Autodesk Inventor part; units mm, degrees
ref_plane "YZ Plane" through (0, 0, 0) normal (1, 0, 0) x (0, 1, 0)
ref_plane "XZ Plane" through (0, 0, 0) normal (0, 1, 0) x (-1, 0, 0)
ref_plane "XY Plane" through (0, 0, 0) normal (0, 0, 1) x (1, 0, 0)
sketch "Sketch1" plane through (0, 0, 0) normal (0, 0, 1) x (1, 0, 0)
  line L0 (-750, 50) -> (750, 50)
  line L1 (750, 50) -> (750, 0)
  line L2 (750, 0) -> (-750, 0)
  line L3 (-750, 0) -> (-750, 50)
  point P0 (0, 0)
  point P1 (0, 0)
  dimension "d0" = 1500
  dimension "d1" = 50
extrude "Plate1" add sketch "Sketch1" along normal blind 2
sketch "Sketch2" plane through (750, 2, 0) normal (0, -1, 0) x (1, 0, 0)
  line L0 (-1500, 0) -> (0, 0)
  line L1 (0, 0) -> (0, 30)
  line L2 (0, 30) -> (-1500, 30)
  line L3 (-1500, 30) -> (-1500, 0)
edge flange "Flange1" height 30 angle 90 thickness 2 bend radius 2.75 thickness toward (0, -1, 0) relief round relief width 2 relief depth 1 edges at (0, 0, 2) wall of the first edge with corners at (-750, 2, 0) (750, 2, 0) (750, 2, 30) (-750, 2, 30)
bend "Bend1"
corner "Corner1"
sketch "Sketch5" plane through (0, 0, 0) normal (0, 0, -1) x (-1, 0, 0)
  line L0 (750, 50) -> (-750, 50)
  line L1 (-1, 30) -> (-1, 50)
  line L2 (750, 0) -> (-750, 0)
  line L3 (-1, 30) -> (1, 30)
  line L4 (1, 30) -> (1, 50)
  point P0 (0, 0)
  point P1 (0, 30)
  point P2 (0, 0)
  dimension "d27" = 2
  dimension "d28" = 30
extrude "Extrusion1" cut sketch "Sketch5" against normal through all
pattern_linear "Rectangular Pattern1" count 3 spacing 500 along (1, 0, 0) of "Extrusion1" first direction both ways yes
sketch "Sketch6" plane through (0, 0, 0) normal (0, 0, -1) x (-1, 0, 0)
  line L0 (-750, 50) -> (-750, 4.75)
  circle A0 centre (-750, 50) radius 22.5
  line L1 (-750, 50) -> (750, 50)
  line L2 (-1, 50) -> (-1, 30)
  line L3 (-499, 50) -> (-499, 30)
  line L4 (-1, 30) -> (-499, 30) construction
  circle A1 centre (-250, 50) radius 22.5
  point P0 (0, 0)
  point P1 (-727.5, 50)
  point P2 (-750, 27.5)
  point P3 (-250, 30)
  dimension "d24" = 45
extrude "Extrusion2" cut sketch "Sketch6" along normal mid plane 30 contours L1 A0 L0 | A1 L1 | L1 A1 picked at (-748.3311, 35.188)
mirror "Mirror1" about plane through (0, 0, 0) normal (1, 0, 0) of "Extrusion2"
sketch "Sketch7" plane through (0, 0, 2) normal (0, 0, 1) x (1, 0, 0)
  line L0 (494, 45) -> (494, 33) construction
  line L1 (494, 33) -> (294, 33) construction
  line L2 (294, 33) -> (294, 45) construction
  line L3 (294, 45) -> (494, 45) construction
  line L4 (272.5, 50) -> (499, 50)
  point P0 (0, 0)
  dimension "d29" = 200
  dimension "d30" = 12
  dimension "d31" = 5
  dimension "d32" = 5
mark "Mark1"
equation "\"d1\" = Стрингер_7"
equation "\"d27\" = d18"
equation "\"d2\" = Thickness"
equation "\"d3\" = BendReliefWidth"
equation "\"d4\" = BendReliefDepth"
equation "\"d5\" = MinimumRemnant"
equation "\"d6\" = TransitionRadius"
equation "\"d9\" = BendRadius"
equation "\"d10\" = CornerReliefSize"
equation "\"d11\" = GapSize"
equation "\"d12\" = JacobiRadiusSize"
equation "\"GapSize\" = Thickness"
equation "\"MinimumRemnant\" = 2 * Thickness"
equation "\"BendReliefDepth\" = 0.5 * Thickness"
equation "\"BendReliefWidth\" = Thickness"
equation "\"CornerReliefSize\" = 4 * Thickness"
equation "\"JacobiRadiusSize\" = BendRadius"
equation "\"TransitionRadius\" = BendRadius"
equation "\"d18\" = Thickness"
properties part number "MSC 057 stringer belly" material "Stainless Steel"
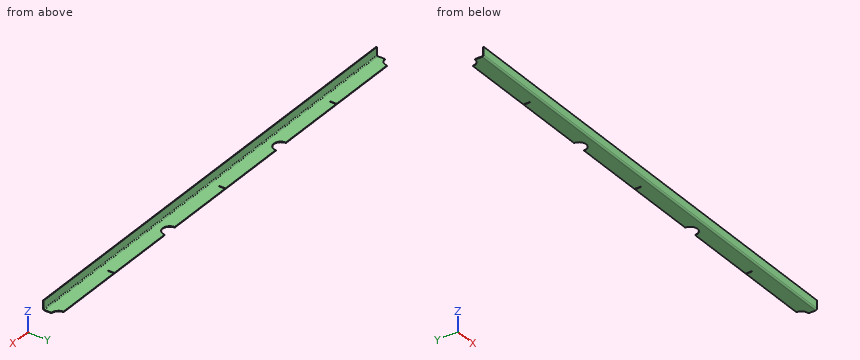
Here's how the part is built. I have some questions about the finished solid (model axes, mm). Coordinates: 2 decimals unless noted, no trailing zeros. Write each loop counter-clockwise with the first axis right and the second up, starting at its lowest first coordinate (ties: lowest second). Pieces come first, ordered by that corner, then holes.
Item 1: If I drill on line 1 (Z direction, x = 33.5, y = 34.5); line 2 (Y direction, x = -122.5, z = 4.5); line 3 (Y direction, x = 302.5, z = 1), over which ranges is the centre line in solid material (lowest first)?
Item 2: I want a section at D-D on x = -250. Write out the boundary of the cut face in (y, z), and give its area (3 significant figures).
Item 3: Will these pins go through, and if not, where does the flat tip stop? pin 1 (10 mm diameter, centred on x = 223.5, z = 17.5, fed in from +Y); pin 2 (1 mm diameter, centred on y = 40, z = 1.5, fed in from +X); pin 3 (2 mm diameter, centred on y = 42.5, z = 1.5, fed in from -X).
Item 4: I want a section at C-C on z = 14.5. Write out the boundary of the cut face in (x, y), and give its area (3 significant figures).
Item 5: I want a section at A-A on x = -406. Write out the boundary of the cut face in (y, z), and give its area (3 significant figures).
Item 6: I want a section at B-B on y = 41.5. Write out the boundary of the cut face in (x, z).
Findings below:
1. line 1: z = 0 to 2
1. line 2: y = 0.01 to 2.01
1. line 3: y = 1.83 to 50
2. outline: (0, 4.75) arc R4.75 ccw to (4.75, 0) - (27.5, 0) - (27.5, 2) - (4.75, 2) arc R2.75 cw to (2, 4.75) - (2, 30) - (0, 30) - close
2. area: 108 mm2
3. pin 1: stops at y = 2
3. pin 2: stops at x = 730.1
3. pin 3: stops at x = -729.17
4. outline: (-750, 0) - (750, 0) - (750, 2) - (-750, 2) - close
4. area: 3,000 mm2
5. outline: (0, 4.75) arc R4.75 ccw to (4.75, 0) - (50, 0) - (50, 2) - (4.75, 2) arc R2.75 cw to (2, 4.75) - (2, 30) - (0, 30) - close
5. area: 153 mm2
6. outline: (-729.17, 0) - (-501, 0) - (-501, 2) - (-729.17, 2) - close; (-499, 0) - (-270.83, 0) - (-270.83, 2) - (-499, 2) - close; (-229.17, 0) - (-1, 0) - (-1, 2) - (-229.17, 2) - close; (1, 0) - (229.17, 0) - (229.17, 2) - (1, 2) - close; (270.83, 0) - (499, 0) - (499, 2) - (270.83, 2) - close; (501, 0) - (729.17, 0) - (729.17, 2) - (501, 2) - close
